```python
from build123d import *

# Parameters (mm, degrees)
SKETCH1_W           = 101.6
SKETCH1_H           = 33.59912
BOSS_EXTRUDE1_DEPTH = 5
SKETCH2_R           = 3.4
SKETCH2_R_2         = 1.9
CUT_EXTRUDE1_DEPTH  = 5
SKETCH5_W           = 15
SKETCH5_H           = 16
CUT_EXTRUDE4_DEPTH  = 5
SKETCH7_W           = 56
SKETCH7_H           = 33.59912
SKETCH7_R           = 1.9
BOSS_EXTRUDE2_DEPTH = 2.1


with BuildPart() as part:
    # Sketch1 → Boss-Extrude1 (new body)
    with BuildSketch(Plane.XY):
        Rectangle(SKETCH1_W, SKETCH1_H)
    extrude(amount=BOSS_EXTRUDE1_DEPTH)

    # Sketch2 → Cut-Extrude1 (cut)
    with BuildSketch(Plane(origin=(0, 0, 0), x_dir=(-1, 0, 0), z_dir=(0, 0, -1))):
        with Locations((40.8, 8.20044)):
            Circle(SKETCH2_R)
        with Locations((21.75, 8.20044)):
            Circle(SKETCH2_R)
        with Locations((-17.4, 1.20044)):
            Circle(SKETCH2_R_2)
        with Locations((-42.8, 1.20044)):
            Circle(SKETCH2_R_2)
    extrude(amount=-CUT_EXTRUDE1_DEPTH, mode=Mode.SUBTRACT)

    # Sketch5 → Cut-Extrude4 (cut)
    with BuildSketch(Plane(origin=(0, 0, 0), x_dir=(-1, 0, 0), z_dir=(0, 0, -1))):
        with Locations((43.3, -8.79956)):
            Rectangle(SKETCH5_W, SKETCH5_H)
    extrude(amount=-CUT_EXTRUDE4_DEPTH, mode=Mode.SUBTRACT)

    # Sketch7 → Boss-Extrude2 (add)
    with BuildSketch(Plane.XY.offset(5)):
        with Locations((22.8, 0)):
            Rectangle(SKETCH7_W, SKETCH7_H)
        with Locations(Location((17.4, 1.20044, 0), (0, 0, 180))):
            Circle(SKETCH7_R, mode=Mode.SUBTRACT)
        with Locations(Location((42.8, 1.20044, 0), (0, 0, 180))):
            Circle(SKETCH7_R, mode=Mode.SUBTRACT)
    extrude(amount=BOSS_EXTRUDE2_DEPTH)


solid = part.part
```
Can you work these out from the model? Positions are in its coordinate system, mm. A direction names the side the tool comes from. Give positions to 0.01 mm unless a question says otherwise; leave off trailing zeros. Loops run counter-clockwise (first coordinate to the right, second up) from the corner with the lowest first, then second, coordinate; pieces in that order, holes last. Notation, with made-up numbers: M 30,8 L 47,8 A27 ccw 47,39 Z; hole C 30,51.5 d6. An arc over 180 degrees is marked long. One line per question, with ' | ' between items. Start each with the question number.
Q1. If we section it at C-C (y = -4.5): Please give me the cut outline in (x, z), plus the area to 3 significant figures.
Q2. If we section it at B-B (z = 3.75): Please give me the cut outline in (x, y), plus the area to 3 significant figures.
Q3. If we mould it in two halves opening along X, with no side actions, what happens to faces 1 (the cylindrical face through (-25, 9.2, 2.5)), 2 (the flat face through (-50.8, 8, 2)), 3 (the flat face through (-43, -0.8, 2))? For each: +X half, -X half, draft (parallel to the pull), parting line (faces both ways), or undercut.
Q4. For faces 4 (the flat face through (-35.8, -9, 2)), 5 (the cylindrical face through (-43.94, 6.9, 2.46)), 6 (the flat face through (-5.2, 0, 6)), which set-ups out of +Z, -Z, +X, -X, +Y, -Y let a thin tool reach every point of the face, with its end or its side?
Q5. For pin 1 Ø8 at (x, y) = (32, -8.5) entering from -Z; pin 2 Ø0.6 at (y, z) = (7, 6.5) entering from -X; pin 3 Ø1.5 at (x, z) = (-41.5, 2.5) entering from -Y; pin 4 Ø11 at (x, y) = (-40.8, 8.2) entering from +Z, each with a flat end and sliding along its axis, tell me the tip position at first contact or that it passes through.
Q6. If I drill on line 1 (Y direction, x = -21.75, z = 3.6); line 2 (X direction, y = 11, z = 1.5); line 3 (Y direction, x = -40.8, z = 3.5), over which ranges is the centre line in solid material (lowest first)? Write a range as from..to.
Q7. If we section it at D-D (x = -21.75): Please give me the cut outline in (y, z).
Q8. If we section it at A-A (x = 42.8): Please give me the cut outline in (y, z).
Computed:
1) outline: M -35.8,0 L 50.8,0 L 50.8,7.1 L -5.2,7.1 L -5.2,5 L -35.8,5 Z | area: 551 mm²
2) outline: M -50.8,-0.8 L -35.8,-0.8 L -35.8,-16.8 L 50.8,-16.8 L 50.8,16.8 L -50.8,16.8 Z; hole C -40.8,8.2 d6.8; hole C -21.75,8.2 d6.8; hole C 17.4,1.2 d3.8; hole C 42.8,1.2 d3.8 | area: 3,080 mm²
3) face 1: undercut | face 2: -X half | face 3: draft
4) face 4: +Z, -Z, -X, -Y | face 5: +Z, -Z | face 6: +Z, -X, +Y, -Y
5) pin 1: stops at z = 0 | pin 2: stops at x = -5.2 | pin 3: stops at y = -0.8 | pin 4: stops at z = 5
6) line 1: y = -16.8..4.8, 11.6..16.8 | line 2: x = -50.8..-42.73, -38.87..-23.68, -19.82..50.8 | line 3: y = -0.8..4.8, 11.6..16.8
7) outline: M -16.8,0 L 4.8,0 L 4.8,5 L -16.8,5 Z; M 11.6,0 L 16.8,0 L 16.8,5 L 11.6,5 Z
8) outline: M -16.8,0 L -0.7,0 L -0.7,7.1 L -16.8,7.1 Z; M 3.1,0 L 16.8,0 L 16.8,7.1 L 3.1,7.1 Z
